Design review of the part built by this model. Coordinates are the model's own, in mm. A direction names the side the tool comes from. Give positions to 0.01 mm unless a question says otherwise; leave off trailing zeros. Write each loop counter-clockwise with the first axis right and the second up, starting at its lowest first coordinate (ties: lowest second). Pieces come first, ordered by that corner, then holes. Notation, with made-up numbers: (14.5, 21.25) -> (32.5, 21.25) arc R28 ccw to (32.5, 60.25) -> close; hole circle Ø6 at (-23.75, 58). An arc over 180 degrees is marked (long way). Answer as a JSON object with one key per item and string values.
```python
from build123d import *

# Parameters (mm, degrees)
SKETCH1_R                                       = 39
BOSS_EXTRUDE1_DEPTH                             = 15
CBORE_FOR_M4_SOCKET_HEAD_CAP_SCREW1_D           = 4.5
CBORE_FOR_M4_SOCKET_HEAD_CAP_SCREW1_CBORE_D     = 8
CBORE_FOR_M4_SOCKET_HEAD_CAP_SCREW1_CBORE_DEPTH = 4
CHAMFER1_SIZE                                   = 1


with BuildPart() as part:
    # Sketch1 → Boss-Extrude1 (new body)
    with BuildSketch(Plane(origin=(0, 0, 0), x_dir=(1, 0, 0), z_dir=(0, 1, 0))):
        Circle(SKETCH1_R)
    extrude(amount=BOSS_EXTRUDE1_DEPTH)

    # CBORE for M4 Socket Head Cap Screw1 (through all)
    with Locations(Plane(origin=(0, 15, 0), x_dir=(-1, 0, 0), z_dir=(0, 1, 0))):
        with Locations((21.213203436, -21.213203436), (21.213203436, 21.213203436), (-21.213203436, 21.213203436), (-21.213203436, -21.213203436)):
            CounterBoreHole(CBORE_FOR_M4_SOCKET_HEAD_CAP_SCREW1_D / 2, CBORE_FOR_M4_SOCKET_HEAD_CAP_SCREW1_CBORE_D / 2, CBORE_FOR_M4_SOCKET_HEAD_CAP_SCREW1_CBORE_DEPTH)

    # Chamfer1
    chamfer1_edges = [part.edges().sort_by_distance(p)[0] for p in [
        (-39, 15, 0),
    ]]
    chamfer(chamfer1_edges, length=CHAMFER1_SIZE)


solid = part.part
```
(1) We need section A-A, the plane x = -21. Give the number of separate pieces and of enclosed holes in the cut face, then the cut area to 3 significant figures.
Here are the results:
{"separate pieces": "3", "enclosed holes": "0", "area": "822 mm²"}
(2) For line 1 along Z through (x, y) = (20, 6.5); line 2 along X through (y, z) = (12.75, 19); line 3 along Z through (x, y) = (23, 11.75), list the stretches that pass through material, from the lowest coordinate up.
Here are the results:
{"line 1": "z = -33.48 to -23.11, -19.32 to 19.32, 23.11 to 33.48", "line 2": "x = -34.06 to -24.55, -17.88 to 17.88, 24.55 to 34.06", "line 3": "z = -31.5 to -24.79, -17.63 to 17.63, 24.79 to 31.5"}
(3) Clearance check with flat-ended pins moving along their axes: pin 1 (6.5 mm diameter, centred on x = 21, z = -23, fed in from +Y); pin 2 (6 mm diameter, centred on x = 20.5, y = 7.5, fed in from -Z); pin 3 (5 mm diameter, centred on x = 21.21, z = -21.21, fed in from +Y); pin 4 (1.5 mm diameter, centred on x = 3, y = 9.5, fed in from -Z). State where each tip first meets the part, or that it passes through.
Here are the results:
{"pin 1": "stops at y = 15", "pin 2": "stops at z = -34.85", "pin 3": "stops at y = 11", "pin 4": "stops at z = -38.94"}
(4) The part is to be moulded in two halves that separate along X. For faces 1 (the cylindrical face through (-21.7, 5.42, -23.41)), 2 (the cylindrical face through (-5.077, 6.902, -38.668)), 3 (the flat face through (-1, 15, -1)), say which applies: +X half, -X half, draft (parallel to the pull), parting line (faces both ways), or undercut.
Here are the results:
{"face 1": "undercut", "face 2": "parting line", "face 3": "draft"}
(5) We need section B-B, the plane y = 3. State the section outline as (x, z) points.
Here are the results:
{"outline": "circle Ø78 at (0, 0); hole circle Ø4.5 at (-21.21, -21.21); hole circle Ø4.5 at (-21.21, 21.21); hole circle Ø4.5 at (21.21, -21.21); hole circle Ø4.5 at (21.21, 21.21)"}
(6) For faces 4 (the cylindrical face through (19.43, 5.42, 19.84)), 5 (the cylindrical face through (24.39, 13.03, 18.78)), list the 3-axis set-ups (+Z, -Z, +X, -X, +Y, -Y) from which the entire face can be reached by the end or side of a thin tool; tool diameter is ignored.
Here are the results:
{"face 4": "+Y, -Y", "face 5": "+Y"}
